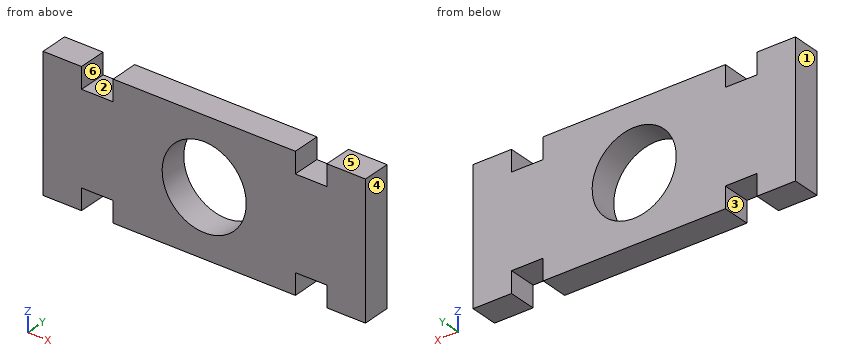
from build123d import *

# Parameters (mm, degrees)
SKETCH_1_R      = 6
EXTRUDE_1_DEPTH = 4


with BuildPart() as part:
    # ｽｹｯﾁ1 → ﾎﾞｽ - 押し出し1 (new body)
    with BuildSketch(Plane(origin=(0, 0, 0), x_dir=(1, 0, 0), z_dir=(0, 1, 0))):
        Polygon((0, 0), (-5.5, 0), (-5.5, 3), (-10, 3), (-10, 0), (-36, 0), (-36, 3), (-40.5, 3), (-40.5, 0), (-46, 0), (-46, 19), (-40.5, 19), (-40.5, 16), (-36, 16), (-36, 19), (-10, 19), (-10, 16), (-5.5, 16), (-5.5, 19), (0, 19), align=None)
        with Locations(Location((-23, 9.5, 0), (0, 0, 270))):
            Circle(SKETCH_1_R, mode=Mode.SUBTRACT)
    extrude(amount=EXTRUDE_1_DEPTH)


solid = part.part
Can you work these out from the model? Positions are in its coordinate system, mm. Face numbers are marked on the shaded views. A direction names the side the tool comes from. Give positions to 0.01 mm unless a question says otherwise; leave off trailing zeros. Loops run counter-clockwise (first coordinate to the right, second up) from the corner with the lowest first, then second, coordinate; pieces in that order, holes last. Notation, with made-up numbers: (55, 24.25) -> (96, 24.25) arc R12 ccw to (96, 30.25) -> close; hole circle Ø4 at (80.5, -28). An arc over 180 degrees is marked (long way). Use one line per item in the form item = value.
1) I need wall thicknesses on line 1 along X through (y, z) = (2.7, -2.75); line 2 along X through (y, z) = (0.95, -9.5); line 3 along Z through (x, y) = (-39, 1.7). Which ranges of each line are inside material? Lowest first, please.
Answers:
line_1 = -46 to -40.5, -36 to -10, -5.5 to 0
line_2 = -46 to -29, -17 to 0
line_3 = -16 to -3
2) For the marked faces 1, 2 and 3, which set-ups out of +Z, -Z, +X, -X, +Y, -Y let a thin tool reach every point of the face, with its end or its side?
Answers:
face_1 = +Z, -Z, -X, +Y, -Y
face_2 = +Z, +Y, -Y
face_3 = -Z, +Y, -Y
3) We'd pull the mould along X, two halves only. Please class the marked faces 4, 5 and 6: released by +X, released by -X, zero draft, split by the parting line, or undercut.
Answers:
face_4 = released by +X
face_5 = zero draft
face_6 = undercut
4) If we section it at C-C (x = -23): Please give me the cut outline in (y, z).
Answers:
outline = (0, -19) -> (4, -19) -> (4, -15.5) -> (0, -15.5) -> close; (0, -3.5) -> (4, -3.5) -> (4, 0) -> (0, 0) -> close
5) If we section it at D-D (y = 2.2): Please give me the cut outline in (x, z), plus the area to 3 significant figures.
Answers:
outline = (-46, -19) -> (-40.5, -19) -> (-40.5, -16) -> (-36, -16) -> (-36, -19) -> (-10, -19) -> (-10, -16) -> (-5.5, -16) -> (-5.5, -19) -> (0, -19) -> (0, 0) -> (-5.5, 0) -> (-5.5, -3) -> (-10, -3) -> (-10, 0) -> (-36, 0) -> (-36, -3) -> (-40.5, -3) -> (-40.5, 0) -> (-46, 0) -> close; hole circle Ø12 at (-23, -9.5)
area = 707 mm²
6) Will this pin go through, and if not, where does the flat tip stop? pin 1 (1.2 mm diameter, centred on x = -38.5, y = 1, fed in from -Z).
Answers:
pin_1 = -16
7) If we section it at B-B (z = -9.5): Please give me the cut outline in (x, y), plus the area to 3 significant figures.
Answers:
outline = (-46, 0) -> (-29, 0) -> (-29, 4) -> (-46, 4) -> close; (-17, 0) -> (0, 0) -> (0, 4) -> (-17, 4) -> close
area = 136 mm²
8) If we section it at A-A (z = -2): Please give me the cut outline in (x, y), plus the area to 3 significant figures.
Answers:
outline = (-46, 0) -> (-40.5, 0) -> (-40.5, 4) -> (-46, 4) -> close; (-36, 0) -> (-10, 0) -> (-10, 4) -> (-36, 4) -> close; (-5.5, 0) -> (0, 0) -> (0, 4) -> (-5.5, 4) -> close
area = 148 mm²
